Can you work these out from the model? Positions are in its coordinate system, mm. A direction names the side the tool comes from. Round coordinates to 2 decimals unless told otherwise and drop trailing zeros. Write each loop counter-clockwise with the first axis right and the second up, starting at its lowest first coordinate (ties: lowest second). Pieces come first, ordered by that corner, then holes. Notation, with made-up numbers: M 63.25,-18 L 100.25,-18 A15 cw 100.25,-11 Z; hole C 34.5,-28 d1. An arc over 180 degrees is marked long. Answer in a Markdown table with one row per item. Add a question column.
(1) If we mould it in two halves opening along Z, with no side actions, what happens to faces 1 (the face through (-0.1, 2.8, 3.5)), 2 (the face through (2.85, 2.77, -6.51)), 3 (the face through (0, 0, -5)), 4 (the face through (-0.047, 0.752, -13.137))? For each: released by +Z, released by -Z, zero draft, split by the parting line, or undercut.
(2) For faces 5 (the face through (0, 1.5, -8)), 6 (the face through (3, 4, -7)), 7 (the face through (-1, 5.9, -17)), 8 (the face through (0.1, 0.8, -3.5)), 9 (the face through (0, 2.5, -16.5)), which set-ups out of +Z, -Z, +X, -X, +Y, -Y let a thin tool reach every point of the face, with its end or its side?
(3) I'm going to push flat-ended pins straight in: pin 1 (2.5 mm diameter, centred on x = -1, z = -6, fed in from +Y); pin 2 (1.5 mm diameter, centred on x = -1, y = 5, fed in from -Z); pin 3 (3 mm diameter, centred on x = 2.5, y = 4, fed in from -Z). Where does each tip first touch, or does it pass through?
(4) Suppose I cut it at B-B, the plane z = 0. Write out the boundary of the cut face in (x, y), then the cut area to 3 significant figures.
(5) Suppose I cut it at A-A, the plane x = 0. Count the separate pieces of the cut face and the enclosed holes in it, then the cut area to 3 significant figures.
(6) If I drill on probe 1 along Z at (x, y) = (0, 3.4) (3 decimals); probe 2 along X at (y, z) = (3.35, 0); probe 3 along X at (y, z) = (5.35, -17.85) (3 decimals), over which ranges is the centre line in solid material (lowest first)?
(7) Suppose I cut it at C-C, the plane y = 3.25. Write out the boundary of the cut face in (x, z) (3 decimals).
Autodesk Inventor part; units mm, degrees
ref_plane "YZ Plane" through (0, 0, 0) normal (1, 0, 0) x (0, 1, 0)
ref_plane "XZ Plane" through (0, 0, 0) normal (0, 1, 0) x (-1, 0, 0)
ref_plane "XY Plane" through (0, 0, 0) normal (0, 0, 1) x (1, 0, 0)
sketch "Эскиз1" plane through (0, 0, 0) normal (0, 1, 0) x (-1, 0, 0)
  circle A0 centre (0, 0) radius 4
  dimension "d0" = 8
extrude "Выдавливание1" add sketch "Эскиз1" along normal blind 4
sketch "Эскиз5" plane through (0, 4, 0) normal (0, 1, 0) x (1, 0, 0)
  circle A0 centre (0, 0) radius 4
  line L0 (-4, 0) -> (4, 0)
  line L1 (4, 0) -> (4, 17.85)
  line L2 (4, 17.85) -> (-4, 17.85)
  line L3 (-4, 17.85) -> (-4, 0)
  circle A1 centre (0, 0) radius 4
  circle A2 centre (0, 17.85) radius 3
  line L4 (4, 0) -> (3, 17.85)
  line L5 (-4, 0) -> (-3, 17.85)
  point P0 (4, 0)
  point P1 (-3.975, 0.4468)
  point P2 (3.975, 0.4468)
  dimension "d27" = 17.85
  dimension "d59" = 6
extrude "Выдавливание4" add sketch "Эскиз5" against normal blind 4 contours L5 A2 L4 A0 | A2 L2 | L2 A2
sketch "Эскиз9" plane through (0, 4, 0) normal (0, -1, 0) x (1, 0, 0)
  circle A0 centre (0, 0) radius 3.5
  line L0 (3.5, 0) -> (-3.5, 0)
  line L1 (3.5, 0) -> (2.25, -12.5)
  line L2 (-3.5, 0) -> (-2.25, -12.5)
  line L3 (2.25, -12.5) -> (-2.25, -12.5)
  point P0 (0, -12.5)
  point P1 (-3.4307, -0.6931)
  point P2 (3.4307, -0.6931)
  dimension "d43" = 7
  dimension "d44" = 4.5
  dimension "d45" = 12.5
extrude "Выдавливание7" cut sketch "Эскиз9" along normal blind 2.5
sketch "Эскиз10" plane through (0, 1.5, 0) normal (0, 1, 0) x (1, 0, 0)
  line L0 (2.25, 12.5) -> (3.4307, 0.6931)
  line L1 (-3.4307, 0.6931) -> (-2.25, 12.5)
  arc A0 (-3.4307, 0.6931) -> (3.4307, 0.6931) centre (0, 0) ccw
  arc A1 (-3.4307, 0.6931) -> (3.4307, 0.6931) centre (0, 0) ccw
  circle A2 centre (0, 0) radius 3.5
  line L2 (-2.25, 12.5) -> (2.25, 12.5)
  point P0 (3.4307, 0.6931)
extrude "Выдавливание8" cut sketch "Эскиз10" against normal through all contours A0 A2
sketch "Эскиз13" plane through (0, 0, 0) normal (0, -1, 0) x (1, 0, 0)
  arc A0 (-3, -17.85) -> (3, -17.85) centre (0, -17.85) ccw
  circle A1 centre (0, -17.85) radius 3
  line L0 (-2.25, -12.5) -> (2.25, -12.5)
  line L1 (-2.25, -12.5) -> (2.25, -12.5)
  line L2 (3.2241, -13.85) -> (-3.2241, -13.85)
  line L3 (-3.2241, -13.85) -> (-3.2241, -20.85)
  line L4 (-3.2241, -20.85) -> (3.2241, -20.85)
  line L5 (3.2241, -20.85) -> (3.2241, -13.85)
  line L6 (-3.975, -0.4468) -> (-3, -17.85)
  line L7 (3, -17.85) -> (3.975, -0.4468)
  point P0 (0, 0)
  point P1 (3, -17.85)
  dimension "d71" = 7
extrude "Выдавливание10" cut sketch "Эскиз13" against normal blind 2.5 contours A1 A0 | L6 L2 L7 A1
sketch "Эскиз14" plane through (0, 2.5, -17.85) normal (0, -1, 0) x (-1, 0, 0)
  arc A0 (3, 0) -> (-3, 0) centre (0, 0) ccw
  line L0 (-3.2241, -4) -> (-3, 0)
  line L1 (3, 0) -> (3.2241, -4)
  line L2 (3.2241, -4) -> (-3.2241, -4)
  point P0 (0, -17.85)
hole "Отверстие4" at (0, 2.5, -17.85) direction (0, 1, 0) diameter 1.95 depth 4
sketch "Эскиз15" plane through (0, 4, 0) normal (0, 1, 0) x (1, 0, 0)
  circle A0 centre (0, 17.85) radius 0.975
  arc A1 (3, 17.85) -> (-3, 17.85) centre (0, 17.85) ccw
  line L0 (3.2241, 13.85) -> (3, 17.85)
  line L1 (-3, 17.85) -> (-3.2241, 13.85)
  line L2 (-3.2241, 13.85) -> (3.2241, 13.85)
  point P0 (0, 0)
extrude "Выдавливание11" add sketch "Эскиз15" along normal blind 1.9
fillet "Сопряжение1" radius 0.95 2 edges at (0, 4, -13.85) (0, 5.9, -13.85)
fillet "Сопряжение2" radius 2.5 1 edges at (0, 0, -13.85)
properties part number "Поворотный рычаг для сервы"
Calculated:
| question | item | result |
|---|---|---|
| 1 | face 1 | undercut |
| 1 | face 2 | undercut |
| 1 | face 3 | zero draft |
| 1 | face 4 | released by -Z |
| 2 | face 5 | +Y |
| 2 | face 6 | +Z, +X, -X, +Y |
| 2 | face 7 | +Z, -Z, +X, -X, +Y |
| 2 | face 8 | +Y, -Y |
| 2 | face 9 | -Z, +X, -X, -Y |
| 3 | pin 1 | y = 1.5 |
| 3 | pin 2 | z = -20.84 |
| 3 | pin 3 | z = -20.68 |
| 4 | outline | M -4,0 L -3.5,0 L -3.5,4 L -4,4 Z; M 3.5,0 L 4,0 L 4,4 L 3.5,4 Z |
| 4 | area | 4.00 mm² |
| 5 | separate pieces | 3 |
| 5 | enclosed holes | 0 |
| 5 | area | 36.7 mm² |
| 6 | probe 1 | -20.85 to -18.825, -16.875 to -12.5, 3.5 to 4 |
| 6 | probe 2 | -4 to -3.5, 3.5 to 4 |
| 6 | probe 3 | -3 to -0.975, 0.975 to 3 |
| 7 | outline | M -3.975,-0.447 L -3,-17.85 A3 ccw 3,-17.85 L 3.975,-0.447 A4 ccw long Z; hole M -3.431,-0.693 L -2.25,-12.5 L 2.25,-12.5 L 3.431,-0.693 A3.5 ccw long Z; hole C 0,-17.85 d1.95 |
